Part model, mm, in its own coordinate system. Face numbers are marked on the shaded views. A direction names the side the tool comes from. Give positions to 0.01 mm unless a question says otherwise; leave off trailing zeros. Order: outer loops, then holes, each group sorted by start corner. A loop starts at its lowest first (then second) coordinate and runs counter-clockwise, first axis right, second up. Notation, with made-up numbers: (14.5, -7) - (28.5, -7) arc R25 cw to (28.5, 27) - close; hole circle Ø4 at (42, 59). An arc over 180 degrees is marked (long way). One line per item, written item: value.
```python
from build123d import *

# Parameters (mm, degrees)
ESQUISSE1_W                                       = 5
ESQUISSE1_H                                       = 40
BOSS_EXTRU_1_DEPTH                                = 20
ESQUISSE1_3_W                                     = 5
ESQUISSE1_3_H                                     = 40
ESQUISSE1_3_W_2                                   = 10
ESQUISSE1_3_H_2                                   = 5
BOSS_EXTRU_2_DEPTH                                = 5
ESQUISSE3_W                                       = 40
ESQUISSE3_H                                       = 5
BOSS_EXTRU_3_DEPTH                                = 20
ENL_V_MAT_EXTRU_2_DEPTH                           = 40
ENL_V_MAT_EXTRU_2_DEPTH_BACK                      = 61
CHAMBRAGE_POUR_VIS_SIX_PANS_CREUX_M41_D           = 4.8
CHAMBRAGE_POUR_VIS_SIX_PANS_CREUX_M41_CBORE_D     = 8
CHAMBRAGE_POUR_VIS_SIX_PANS_CREUX_M41_CBORE_DEPTH = 2
CHAMBRAGE_POUR_VIS_SIX_PANS_CREUX_2_D             = 4.8
CHAMBRAGE_POUR_VIS_SIX_PANS_CREUX_2_CBORE_D       = 8
CHAMBRAGE_POUR_VIS_SIX_PANS_CREUX_2_CBORE_DEPTH   = 2
CHAMBRAGE_POUR_VIS_SIX_PANS_CREUX_3_D             = 4.8
CHAMBRAGE_POUR_VIS_SIX_PANS_CREUX_3_CBORE_D       = 8
CHAMBRAGE_POUR_VIS_SIX_PANS_CREUX_3_CBORE_DEPTH   = 2


with BuildPart() as part:
    # Esquisse1 → Boss.-Extru.1 (new body)
    with BuildSketch(Plane(origin=(0, 0, 0), x_dir=(1, 0, 0), z_dir=(0, 1, 0))):
        with Locations((2.5, 30)):
            Rectangle(ESQUISSE1_W, ESQUISSE1_H)
        Polygon((0, 50), (5, 50), (5, 55), (15, 55), (15, 50), (20, 50), (20, 60), (0, 60), align=None)
        Polygon((15, 5), (5, 5), (5, 10), (0, 10), (0, 0), (20, 0), (20, 10), (15, 10), align=None)
    extrude(amount=BOSS_EXTRU_1_DEPTH)

    # Esquisse1<3> → Boss.-Extru.2 (add)
    with BuildSketch(Plane(origin=(0, 0, 0), x_dir=(1, 0, 0), z_dir=(0, 1, 0))):
        Polygon((0, 50), (5, 50), (5, 55), (15, 55), (15, 50), (20, 50), (20, 60), (0, 60), align=None)
        with Locations((17.5, 30)):
            Rectangle(ESQUISSE1_3_W, ESQUISSE1_3_H)
        with Locations((10, 52.5)):
            Rectangle(ESQUISSE1_3_W_2, ESQUISSE1_3_H_2)
        with Locations((10, 30)):
            Rectangle(ESQUISSE1_3_W_2, ESQUISSE1_3_H)
        with Locations((2.5, 30)):
            Rectangle(ESQUISSE1_3_W, ESQUISSE1_3_H)
        Polygon((15, 5), (5, 5), (5, 10), (0, 10), (0, 0), (20, 0), (20, 10), (15, 10), align=None)
        with Locations((10, 7.5)):
            Rectangle(ESQUISSE1_3_W_2, ESQUISSE1_3_H_2)
    extrude(amount=-BOSS_EXTRU_2_DEPTH)

    # Esquisse3 → Boss.-Extru.3 (add)
    with BuildSketch(Plane.ZY):
        Polygon((-55, 20), (-55, -5), (-50, -5), (-50, 15), (-50, 20), align=None)
        Polygon((-10, 15), (-10, -5), (-5, -5), (-5, 20), (-10, 20), align=None)
        with Locations((-30, 17.5)):
            Rectangle(ESQUISSE3_W, ESQUISSE3_H)
    extrude(amount=BOSS_EXTRU_3_DEPTH)

    # Esquisse4 → Enlèv. mat.-Extru.2 (cut, two sides)
    with BuildSketch(Plane.XY) as enl_v_mat_extru_2_sk:
        with BuildLine():
            ThreePointArc((12.759432597, 9.481134806), (11.573760378, 11.607761826), (9.141398608, 11.717202783))
            Line((9.141398608, 11.717202783), (11.377466586, 7.245066828))
            ThreePointArc((11.377466586, 7.245066828), (12.386059618, 8.166807025), (12.759432597, 9.481134806))
        make_face()
        with BuildLine():
            Line((11.377466586, 7.245066828), (9.141398608, 11.717202783))
            ThreePointArc((9.141398608, 11.717202783), (8.02336462, 8.363100817), (11.377466586, 7.245066828))
        make_face()
    extrude(amount=ENL_V_MAT_EXTRU_2_DEPTH, mode=Mode.SUBTRACT)
    extrude(enl_v_mat_extru_2_sk.sketch, amount=-ENL_V_MAT_EXTRU_2_DEPTH_BACK, mode=Mode.SUBTRACT)

    # Chambrage pour vis à six pans creux M41 (through all)
    with Locations(Plane(origin=(-10, 7.5, -5), x_dir=(0, 1, 0), z_dir=(0, 0, 1))):
        with Locations((0, 0)):
            CounterBoreHole(CHAMBRAGE_POUR_VIS_SIX_PANS_CREUX_M41_D / 2, CHAMBRAGE_POUR_VIS_SIX_PANS_CREUX_M41_CBORE_D / 2, CHAMBRAGE_POUR_VIS_SIX_PANS_CREUX_M41_CBORE_DEPTH)

    # Chambrage pour vis _ six pans creux  2 (through all)
    with Locations(Plane(origin=(-10, 20, -45), x_dir=(0, 0, 1), z_dir=(0, 1, 0))):
        with Locations((0, 0), (30, 0)):
            CounterBoreHole(CHAMBRAGE_POUR_VIS_SIX_PANS_CREUX_2_D / 2, CHAMBRAGE_POUR_VIS_SIX_PANS_CREUX_2_CBORE_D / 2, CHAMBRAGE_POUR_VIS_SIX_PANS_CREUX_2_CBORE_DEPTH)

    # Chambrage pour vis _ six pans creux  3 (through all)
    with Locations(Plane(origin=(-10, 7.5, -55), x_dir=(-1, 0, 0), z_dir=(0, 0, -1))):
        with Locations((0, 0)):
            CounterBoreHole(CHAMBRAGE_POUR_VIS_SIX_PANS_CREUX_3_D / 2, CHAMBRAGE_POUR_VIS_SIX_PANS_CREUX_3_CBORE_D / 2, CHAMBRAGE_POUR_VIS_SIX_PANS_CREUX_3_CBORE_DEPTH)


solid = part.part
```
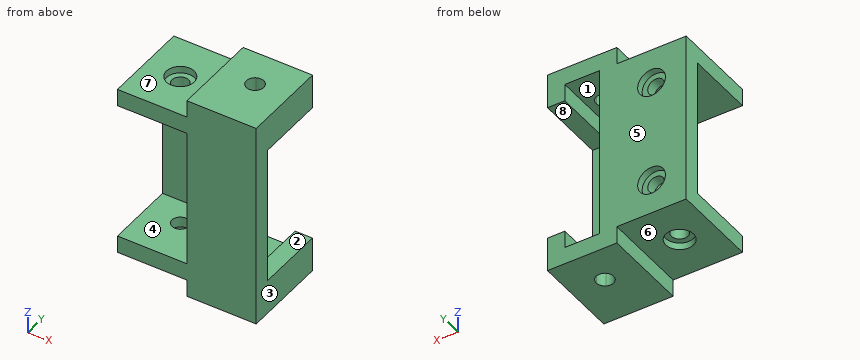
1) Slice it at D-D on x = -10. Count the separate pieces of the cut face and the enclosed holes in it, then the cut area to 3 significant figures.
Answer:
separate pieces: 5
enclosed holes: 0
area: 328 mm2
2) Drop flat-ended pins along their axis: P1, Ø1.5, axis at y = 14.5, z = -26, coming from the +X side; P2, Ø3, axis at x = 9, z = -37.5, coming from the +Y side; P3, Ø6, axis at x = -14, z = -39.5, coming from the -Y side; P4, Ø2, axis at x = 7.5, y = 16.5, coming from the +Z side. Give the stop position or say it passes through.
Answer:
P1: stops at x = 5
P2: stops at y = 0
P3: stops at y = 15
P4: stops at z = 0
3) Slice it at A-A on z = -45. Write the cut outline in (x, y), then the cut area to 3 significant figures.
Answer:
outline: (-20, 15) - (-12.4, 15) - (-12.4, 18) - (-14, 18) - (-14, 20) - (-20, 20) - close; (-7.6, 15) - (0, 15) - (0, -5) - (20, -5) - (20, 0) - (5, 0) - (5, 20) - (-6, 20) - (-6, 18) - (-7.6, 18) - close
area: 270 mm2
4) Wall check: line 1 along X through (y, z) = (7.5, -8.6); line 2 along Z through (x, y) = (-12, -3.5); line 3 along X through (y, z) = (15.8, -45). Give the ranges that are in metal, low to high. Write a range as [from, to].
Answer:
line 1: x = [-20, -12.4], [-7.6, 5], [15, 20]
line 2: z = [-55, -50], [-10, -5]
line 3: x = [-20, -12.4], [-7.6, 5]
5) Slice it at C-C on z = -30. Write the cut outline in (x, y).
Answer:
outline: (-20, 15) - (0, 15) - (0, -5) - (20, -5) - (20, 0) - (5, 0) - (5, 20) - (-20, 20) - close
6) Slice it at B-B on y = 1.5. Write the cut outline in (x, z).
Answer:
outline: (-20, -55) - (0, -55) - (0, -60) - (20, -60) - (20, -50) - (15, -50) - (15, -55) - (5, -55) - (5, -5) - (15, -5) - (15, -10) - (20, -10) - (20, 0) - (0, 0) - (0, -5) - (-20, -5) - (-20, -10) - (0, -10) - (0, -50) - (-20, -50) - close
7) Which spindle directions (+Z, -Z, +X, -X, +Y, -Y) get a long thin tool onto all of the face, cutting with end or side? Do the marked faces 4, 5, 6, 7 and 8. Say none if no direction does.
Answer:
face 4: -X, -Y
face 5: +Z, -Z, +X, -X, +Y
face 6: -Z, -X, +Y, -Y
face 7: +Z, -X, +Y, -Y
face 8: +X, +Y
8) Two-plate mould, pull along X, no slides. Class the marked faces 1, 2 and 3: pulls with the +X half, pulls with the -X half, needs draft (parallel to the pull), parting line crosses it, or undercut.
Answer:
face 1: undercut
face 2: needs draft
face 3: pulls with the +X half
